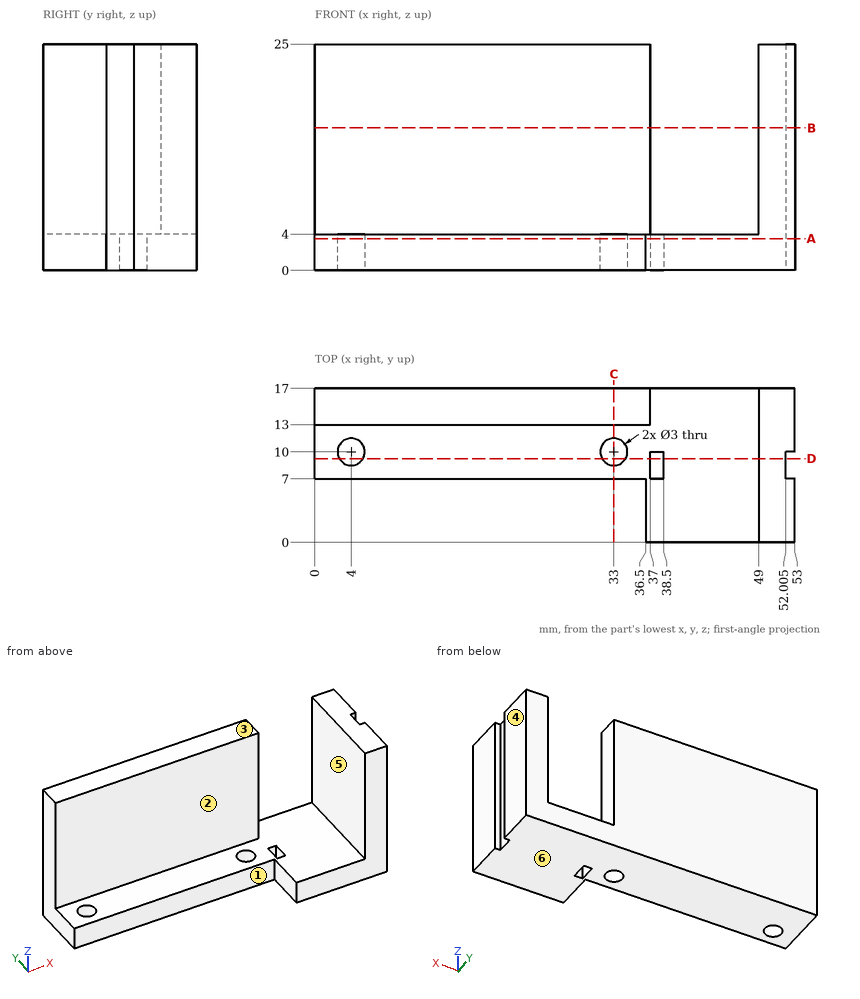
Here's the drawing with two shaded views (mm, measured from the low corner). I have some questions. A direction names the side the tool comes from. Give positions to 0.01 mm unless a question says otherwise; leave off trailing zeros. Loops run counter-clockwise (first coordinate to the right, second up) from the corner with the lowest first, then second, coordinate; pieces in that order, holes last. Notation, with made-up numbers: (-24.5, -14) - (16.5, -14) arc R31 ccw to (16.5, 18) - close; hole circle Ø4 at (-21.5, 70). An arc over 180 degrees is marked (long way). Return JSON: item names as keys, results as strings.
1. For the marked faces 1, 2 and 3, which set-ups out of +Z, -Z, +X, -X, +Y, -Y let a thin tool reach every point of the face, with its end or its side?
Output values:
{"face 1": "+Z, -Z, -X, -Y", "face 2": "+Z, -X, -Y", "face 3": "+Z, +X, -X, +Y, -Y"}
2. I want a section at B-B on z = 15.75. Please give me the cut outline in (x, y) (1 decimal), and give its area (3 significant figures).
Output values:
{"outline": "(0, 13) - (37, 13) - (37, 17) - (0, 17) - close; (49, 0) - (53, 0) - (53, 7) - (52, 7) - (52, 10) - (53, 10) - (53, 17) - (49, 17) - close", "area": "213 mm²"}
3. If I drill on line 1 (Y direction, x = 4, z = 1.8); line 2 (X direction, y = 4.5, z = 4.5); line 3 (Y direction, x = 5, z = 16.5), over which ranges is the centre line in solid material (lowest first)?
Output values:
{"line 1": "y = 7 to 8.5, 11.5 to 17", "line 2": "x = 49 to 53", "line 3": "y = 13 to 17"}
4. I want a section at D-D on y = 9.25. Please give me the cut outline in (x, z) (1 decimal).
Output values:
{"outline": "(0, 0) - (2.7, 0) - (2.7, 4) - (0, 4) - close; (5.3, 0) - (31.7, 0) - (31.7, 4) - (5.3, 4) - close; (34.3, 0) - (37, 0) - (37, 4) - (34.3, 4) - close; (38.5, 0) - (52, 0) - (52, 25) - (49, 25) - (49, 4) - (38.5, 4) - close"}
5. We'd pull the mould along X, two halves only. Please class the marked faces 4, 5 and 6: +X half, -X half, draft (parallel to the pull), parting line (faces both ways), or undercut.
Output values:
{"face 4": "+X half", "face 5": "undercut", "face 6": "draft"}
6. I want a section at A-A on z = 3.5. Please give me the cut outline in (x, y) (1 decimal), and give its area (3 significant figures).
Output values:
{"outline": "(0, 7) - (36.5, 7) - (36.5, 0) - (53, 0) - (53, 7) - (52, 7) - (52, 10) - (53, 10) - (53, 17) - (0, 17) - close; hole circle Ø3 at (4, 10); hole circle Ø3 at (33, 10); hole (37, 7) - (38.5, 7) - (38.5, 10) - (37, 10) - close", "area": "624 mm²"}
7. I'm going to push flat-ended pins straight in: pin 1 Ø1 at (x, y) = (33.5, 7) entering from +Z; pin 2 Ø1.2 at (y, z) = (2.5, 2.5) entering from -X; pin 3 Ø8 at (x, z) = (39, 21) entering from -Y. Where does each tip first touch, or does it pass through?
Output values:
{"pin 1": "stops at z = 4", "pin 2": "stops at x = 36.5", "pin 3": "stops at y = 13"}
8. I want a section at C-C on x = 33. Please give me the cut outline in (y, z).
Output values:
{"outline": "(7, 0) - (8.5, 0) - (8.5, 4) - (7, 4) - close; (11.5, 0) - (17, 0) - (17, 25) - (13, 25) - (13, 4) - (11.5, 4) - close"}
